Here's the drawing with two shaded views (mm, measured from the low corner). I have some questions. Coordinates: 2 decimals unless noted, no trailing zeros. Order: outer loops, then holes, each group sorted by start corner. A loop starts at its lowest first (then second) coordinate and runs counter-clockwise, first axis right, second up. Notation, with made-up numbers: (-40, 45.25) - (3, 45.25) arc R10 cw to (3, 52.25) - close; hole circle Ø10 at (28, -10.75). An arc over 180 degrees is marked (long way). Answer as CSV lines item,"result". Start each with the question number.
1. I want a section at C-C, the plane z = 6.75. List the corners of the cut face in (x, y) for me (3 decimals).
2. I need wall thicknesses on probe 1 along Z at (x, y) = (13.25, 1.45); probe 2 along X at (y, z) = (0.75, 7); probe 3 along X at (y, z) = (1, 13.5). Which ranges of each line are inside material? Lowest first, please.
3. I want a section at B-B, the plane x = 10.16. List the corners of the cut face in (y, z) for me (3 decimals), and give its area (3 significant figures).
4. I want a section at A-A, the plane y = 1.25. List the corners of the cut face in (x, z) for me.
5. For pin 1 (1.5 mm diameter, centred on y = 1.5, z = 14.5, fed in from +X); pin 2 (1.5 mm diameter, centred on x = 13.5, y = 1.5, fed in from +Z), each with a flat end and sliding along its axis, tell me the tip position at first contact or that it passes through.
6. I want a section at D-D, the plane x = 12.25. List the corners of the cut face in (y, z) for me (3 decimals).
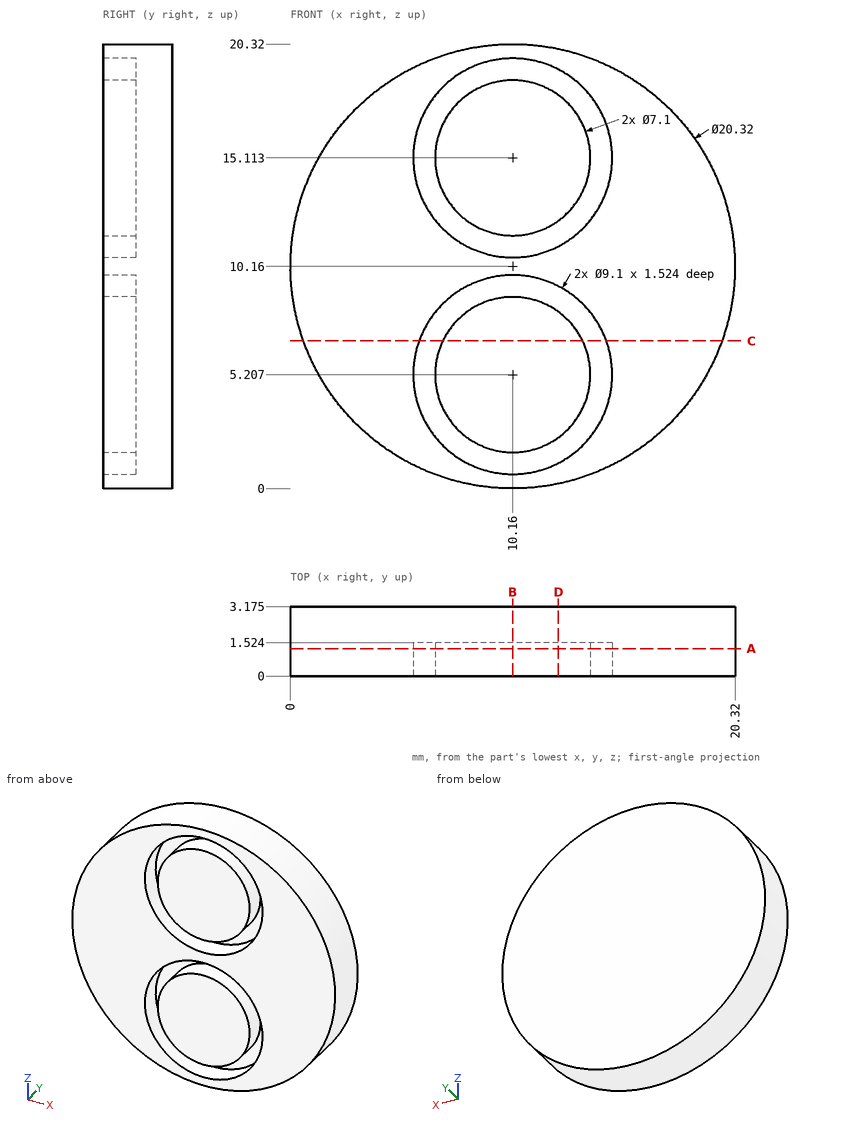
Solved:
1,outline,"(0.589, 0) - (5.88, 0) - (5.88, 1.524) - (6.963, 1.524) - (6.963, 0) - (13.357, 0) - (13.357, 1.524) - (14.44, 1.524) - (14.44, 0) - (19.731, 0) - (19.731, 3.175) - (0.589, 3.175) - close"
2,probe 1,"z = 0.48 to 1.87, 3.46 to 6.95, 8.55 to 11.77, 13.37 to 16.86, 18.45 to 19.84"
2,probe 2,"x = 0.5 to 5.98, 7.1 to 13.22, 14.34 to 19.82"
2,probe 3,"x = 0.56 to 5.91, 7 to 13.32, 14.41 to 19.76"
3,outline,"(0, 0) - (3.175, 0) - (3.175, 20.32) - (0, 20.32) - (0, 19.663) - (1.524, 19.663) - (1.524, 18.663) - (0, 18.663) - (0, 11.563) - (1.524, 11.563) - (1.524, 10.563) - (0, 10.563) - (0, 9.757) - (1.524, 9.757) - (1.524, 8.757) - (0, 8.757) - (0, 1.657) - (1.524, 1.657) - (1.524, 0.657) - (0, 0.657) - close"
3,area,"58.4 mm2"
4,outline,"circle Ø20.32 at (10.16, 10.16); circle Ø7.1 at (10.16, 5.21); circle Ø7.1 at (10.16, 15.11); hole circle Ø9.1 at (10.16, 5.21); hole circle Ø9.1 at (10.16, 15.11)"
5,pin 1,"stops at x = 19.66"
5,pin 2,"stops at z = 19.98"
6,outline,"(0, 0.217) - (3.175, 0.217) - (3.175, 20.103) - (0, 20.103) - (0, 19.155) - (1.524, 19.155) - (1.524, 17.983) - (0, 17.983) - (0, 12.243) - (1.524, 12.243) - (1.524, 11.071) - (0, 11.071) - (0, 9.249) - (1.524, 9.249) - (1.524, 8.077) - (0, 8.077) - (0, 2.337) - (1.524, 2.337) - (1.524, 1.165) - (0, 1.165) - close"
